```python
from build123d import *

# Parameters (mm, degrees)
SKETCH1_W           = 10.67
SKETCH1_H           = 12.88
SKETCH1_R           = 1.855
BOSS_EXTRUDE1_DEPTH = 1.4
SKETCH2_W           = 0.89
SKETCH2_H           = 6.605
CUT_EXTRUDE1_DEPTH  = 2.4
SKETCH3_W           = 0.35
SKETCH3_H           = 1
CUT_EXTRUDE2_DEPTH  = 2.4


with BuildPart() as part:
    # Sketch1 → Boss-Extrude1 (new body)
    with BuildSketch(Plane(origin=(0, 0, 0), x_dir=(1, 0, 0), z_dir=(0, 1, 0))):
        with Locations((0, -3.39)):
            Rectangle(SKETCH1_W, SKETCH1_H)
        Circle(SKETCH1_R, mode=Mode.SUBTRACT)
    extrude(amount=BOSS_EXTRUDE1_DEPTH)

    # Sketch2 → Cut-Extrude1 (cut, through all)
    with BuildSketch(Plane(origin=(0, 1.4, 0), x_dir=(1, 0, 0), z_dir=(0, 1, 0))):
        with Locations((-4.89, -6.5275)):
            Rectangle(SKETCH2_W, SKETCH2_H)
    cut_extrude1 = extrude(amount=-CUT_EXTRUDE1_DEPTH, mode=Mode.SUBTRACT)

    # Mirror1: Cut-Extrude1 across plane
    add(cut_extrude1.mirror(Plane(origin=(0, 0, 0), x_dir=(0, 0, 1), z_dir=(1, 0, 0))), mode=Mode.SUBTRACT)

    # Sketch3 → Cut-Extrude2 (cut, through all)
    with BuildSketch(Plane(origin=(0, 1.4, 0), x_dir=(1, 0, 0), z_dir=(0, 1, 0))):
        with Locations((-4.27, -3.725)):
            Rectangle(SKETCH3_W, SKETCH3_H)
    cut_extrude2 = extrude(amount=-CUT_EXTRUDE2_DEPTH, mode=Mode.SUBTRACT)

    # Mirror2: Cut-Extrude2 across plane
    add(cut_extrude2.mirror(Plane(origin=(0, 0, 0), x_dir=(0, 0, 1), z_dir=(1, 0, 0))), mode=Mode.SUBTRACT)


solid = part.part
```
Geometry check sheet. Reference: the model listing, model coordinates, mm. A direction names the side the tool comes from. Coordinates: 2 decimals unless noted, no trailing zeros. Loops run counter-clockwise (first coordinate to the right, second up) from the corner with the lowest first, then second, coordinate; pieces in that order, holes last. Notation, with made-up numbers: (42.5, 18.25) - (99.5, 18.25) arc R23 ccw to (99.5, 43.25) - close; hole circle Ø6 at (-38.75, 61). An arc over 180 degrees is marked (long way). One line per item, written item: value. Start each with the question number.
(1) Depth check by flat-ended pin: P1, Ø0.8, axis at y = 0.5, z = 4, coming from the -X side (3 decimals); P2, Ø0.8, axis at y = 0.5, z = 4, coming from the +X side (3 decimals); P3, Ø0.6, axis at x = 5, y = 1, coming from the +Z side (3 decimals). Enter the tip coordinate at first touch or a pass-through.
(2) Cross-section at D-D on z = 7. Enter the section's corners in (x, y) (3 decimals).
(3) Material ranges on line 1 (X direction, y = 0.95, z = 0) (3 decimals); line 2 (Z direction, x = 0, y = 0.6) (3 decimals); line 3 (Z direction, x = 4.75, y = 0.35) (3 decimals), recorded low to high. Write a range as [from, to].
(4) Cross-section at B-B on x = 4.25. Enter the section's corners in (y, z) (3 decimals).
(5) Cross-section at C-C on y = 1.15. Enter the section's corners in (x, z) (3 decimals), plus the area to 3 significant figures.
(6) Tool access check on faces 1 (the flat face through (4.445, 1, 7)), 2 (the flat face through (-4.445, 1, 7)), 3 (the flat face through (-5, 1, 3.225)). Record the directions out of +Z, -Z, +X, -X, +Y, -Y that give a thin tool (end or side, any length) a straight path to the whole face; none if there is none.
(7) Mould release check, pull along Z, two halves, no side actions. Record for faces 4 (the flat face through (0, 1, -3.05)), 5 (the flat face through (4.095, 1, 4)), 6 (the flat face through (0, 0, 3)): released by +Z, released by -Z, zero draft, split by the parting line, or undercut.
(8) Cross-section at A-A on z = 0. Enter the section's corners in (x, y) (3 decimals).
Results below:
1. P1: stops at x = -4.445
1. P2: stops at x = 4.445
1. P3: stops at z = 3.225
2. outline: (-4.445, 0) - (4.445, 0) - (4.445, 1.4) - (-4.445, 1.4) - close
3. line 1: x = [-5.335, -1.855], [1.855, 5.335]
3. line 2: z = [-3.05, -1.855], [1.855, 9.83]
3. line 3: z = [-3.05, 3.225]
4. outline: (0, -3.05) - (1.4, -3.05) - (1.4, 3.225) - (0, 3.225) - close; (0, 4.225) - (1.4, 4.225) - (1.4, 9.83) - (0, 9.83) - close
5. outline: (-5.335, -3.05) - (5.335, -3.05) - (5.335, 3.225) - (4.095, 3.225) - (4.095, 4.225) - (4.445, 4.225) - (4.445, 9.83) - (-4.445, 9.83) - (-4.445, 4.225) - (-4.095, 4.225) - (-4.095, 3.225) - (-5.335, 3.225) - close; hole circle Ø3.71 at (0, 0)
5. area: 114 mm2
6. face 1: +Z, +X, +Y, -Y
6. face 2: +Z, -X, +Y, -Y
6. face 3: -X, +Y, -Y
7. face 4: released by -Z
7. face 5: undercut
7. face 6: zero draft
8. outline: (-5.335, 0) - (-1.855, 0) - (-1.855, 1.4) - (-5.335, 1.4) - close; (1.855, 0) - (5.335, 0) - (5.335, 1.4) - (1.855, 1.4) - close
